Can you work these out from the drawing? Everything is in mm from the part's minimum corner. A direction names the side the tool comes from. Round coordinates to 2 decimals unless told otherwise and drop trailing zeros. Loops run counter-clockwise (first coordinate to the right, second up) from the corner with the lowest first, then second, coordinate; pieces in that order, holes last. Notation, with made-up numbers: (-2.75, -10) -> (45.25, -10) arc R32 ccw to (45.25, 19) -> close; hole circle Ø3 at (83.5, 64). An arc over 180 degrees is marked (long way). One line per item, written item: value.
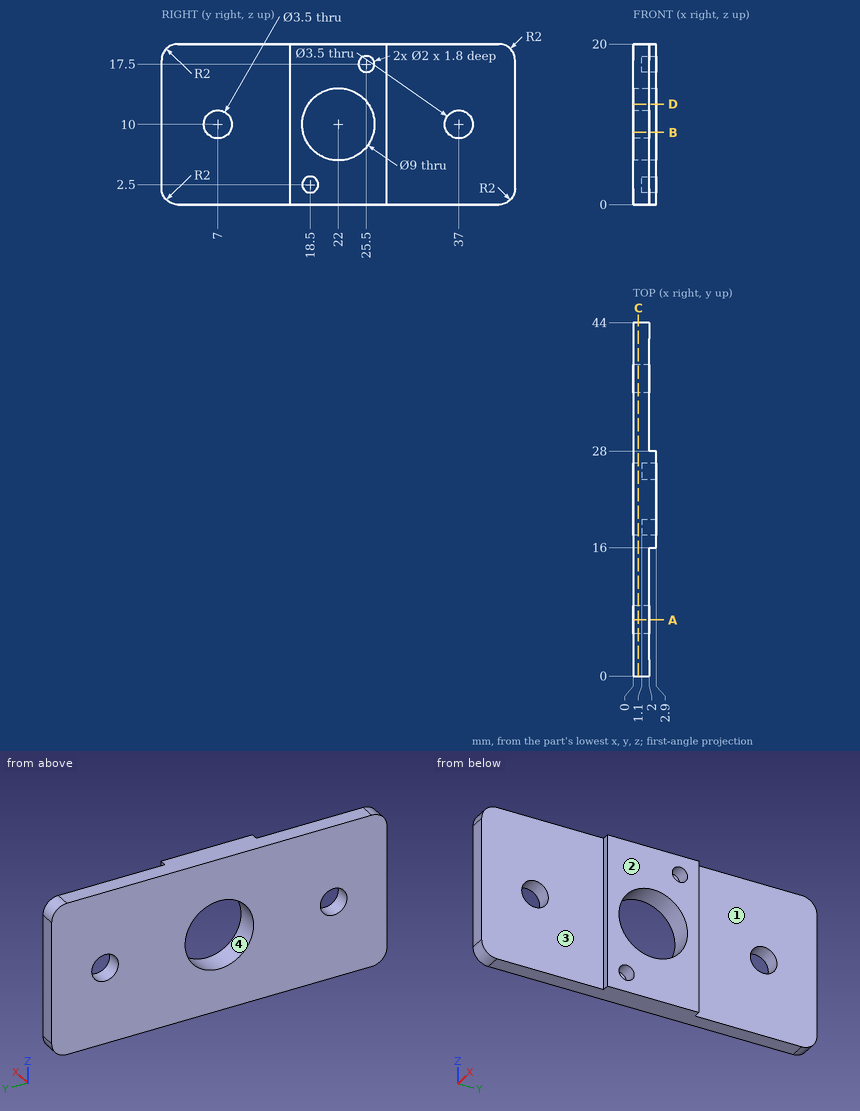
(1) Imagine slicing it at B-B on z = 9. Write out the boundary of the cut face in (x, y).
Results below:
outline: (0, 0) -> (2, 0) -> (2, 5.56) -> (0, 5.56) -> close; (0, 8.44) -> (2, 8.44) -> (2, 16) -> (2.9, 16) -> (2.9, 17.61) -> (0, 17.61) -> close; (0, 26.39) -> (2.9, 26.39) -> (2.9, 28) -> (2, 28) -> (2, 35.56) -> (0, 35.56) -> close; (0, 38.44) -> (2, 38.44) -> (2, 44) -> (0, 44) -> close
(2) Please list where these lines run through material, in increasing order: L1, parallel to Y at x = 1.55, z = 10; L2, parallel to Y at x = 2.3, z = 17.5; L3, parallel to Y at x = 1.5, z = 2.5.
Results below:
L1: y = 0 to 5.25, 8.75 to 17.5, 26.5 to 35.25, 38.75 to 44
L2: y = 16 to 24.5, 26.5 to 28
L3: y = 0 to 17.5, 19.5 to 44
(3) Imagine slicing it at D-D on z = 12.5. Write out the boundary of the cut face in (x, y).
Results below:
outline: (0, 0) -> (2, 0) -> (2, 16) -> (2.9, 16) -> (2.9, 18.26) -> (0, 18.26) -> close; (0, 25.74) -> (2.9, 25.74) -> (2.9, 28) -> (2, 28) -> (2, 44) -> (0, 44) -> close
(4) Imagine slicing it at A-A on y = 7. Write out the boundary of the cut face in (x, z).
Results below:
outline: (0, 0) -> (2, 0) -> (2, 8.25) -> (0, 8.25) -> close; (0, 11.75) -> (2, 11.75) -> (2, 20) -> (0, 20) -> close
(5) We'd pull the mould along Z, two halves only. Please class the marked faces 3 and 4: +Z half, -Z half, draft (parallel to the pull), parting line (faces both ways), or undercut.
Results below:
face 3: draft
face 4: undercut
(6) On a 3-axis mill with a long thin cutter (end or side, diameter ignored), from which of +Z, -Z, +X, -X, +Y, -Y can I reach the whole of each face in a straight line? I mean the marked faces 1 and 2. Say none if no direction works.
Results below:
face 1: +Z, -Z, +X, +Y
face 2: +Z, -Z, +X, +Y, -Y
(7) For pin 1 Ø0.6 at (y, z) = (18.5, 2) entering from +X; pin 2 Ø8 at (y, z) = (9, 8.5) entering from +X; pin 3 Ø3 at (y, z) = (37, 10) entering from +X; pin 4 Ø1 at (y, z) = (26, 17) entering from +X, each with a flat end and sliding along its axis, tell me the tip position at first contact or that it passes through.
Results below:
pin 1: stops at x = 1.1
pin 2: stops at x = 2
pin 3: passes through
pin 4: stops at x = 2.9
(8) Imagine slicing it at C-C on x = 0.65. Write out the boundary of the cut face in (y, z), then the cut area to 3 significant figures.
Results below:
outline: (0, 2) arc R2 ccw to (2, 0) -> (42, 0) arc R2 ccw to (44, 2) -> (44, 18) arc R2 ccw to (42, 20) -> (2, 20) arc R2 ccw to (0, 18) -> close; hole circle Ø3.5 at (7, 10); hole circle Ø9 at (22, 10); hole circle Ø3.5 at (37, 10)
area: 794 mm²
